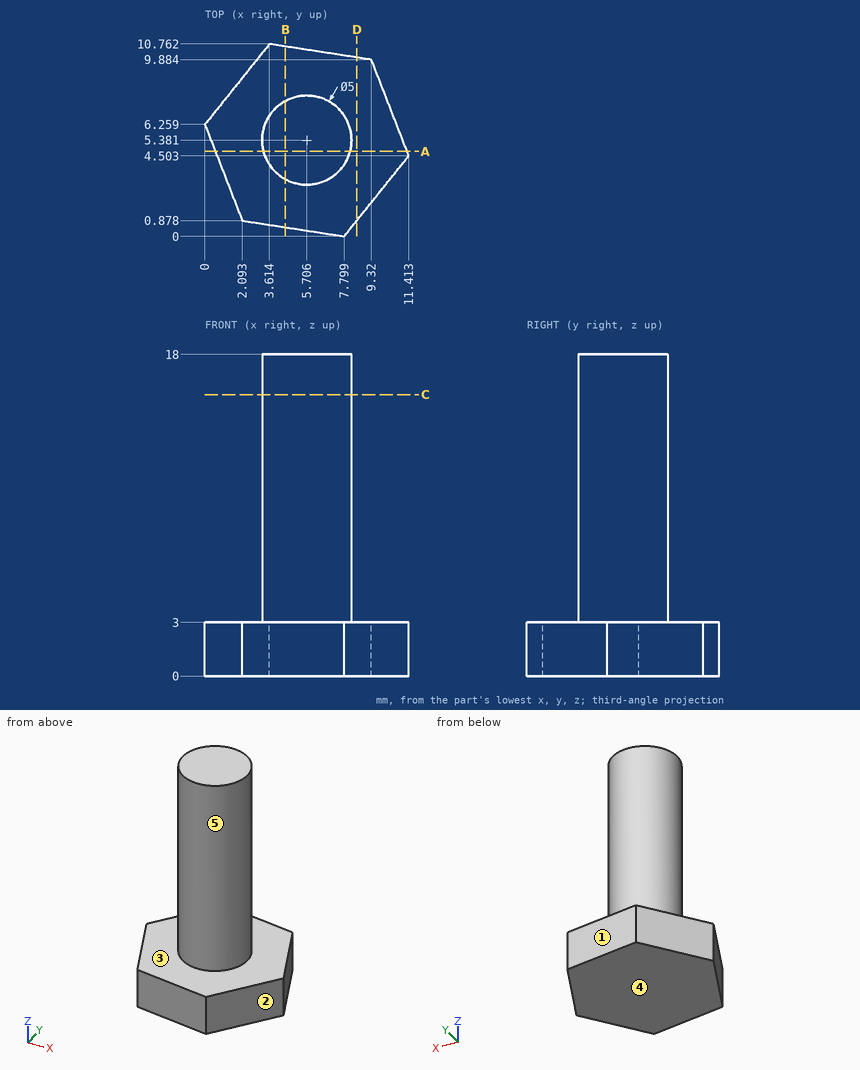
Input: dimensioned drawing with shaded views. Units: mm. Origin: part minimum x, y, z. A direction names the side the tool comes from. Round coordinates to 2 decimals unless told otherwise and drop trailing zeros. Loops run counter-clockwise (first coordinate to the right, second up) from the corner with the lowest first, then second, coordinate; pieces in that order, holes last. Notation, with made-up numbers: M -23,42 L 30,42 A18 cw 30,72 Z; hole C 88.5,78 d2. An arc over 180 degrees is marked long. Answer in a Markdown table with one row per item. Add a question column.
1. Section B-B (x = 4.5). Output: boundary loops of the cut face in (y, z) (1 decimal).
2. Mould query, pull axis Y, two halves, no side actions, for the marked faces 1, 2 and 3. Classes: released by +Y, released by -Y, zero draft, split by the parting line, or undercut.
3. Section D-D (x = 8.5). Output: boundary loops of the cut face in (y, z).
4. Ray query, probe 1 along Z at (x, y) = (9.75, 4); probe 2 along X at (y, z) = (5.5, 7.25); probe 3 along Y at (x, z) = (3.5, 7) (1 decimal). Return the intervals inside material, ascending.
5. Contact query for flat-ended pins moving along their axis: pin 1 (2 mm diameter, centred on y = 8, z = 12, fed in from +X); pin 2 (1.5 mm diameter, centred on x = 8, y = 2, fed in from +Z); pin 3 (1 mm diameter, centred on y = 1.5, z = 3, fed in from -X); pin 4 (1.5 mm diameter, centred on x = 9, z = 8, fed in from +Y). Output: stop coordinate, or through.
6. Section C-C (z = 15.75). Output: boundary loops of the cut face in (x, y), and give its area (3 significant figures).
7. Section A-A (y = 4.75). Output: boundary loops of the cut face in (x, z) (1 decimal).
8. Set-up query: the marked faces 4 and 5. Return all of +Z, -Z, +X, -X, +Y, -Y with unobstructed straight access to the full face (end or side cutting, diameter ignored); none if empty.
Values follow:
| question | item | result |
|---|---|---|
| 1 | outline | M 0.5,0 L 10.6,0 L 10.6,3 L 7.6,3 L 7.6,18 L 3.2,18 L 3.2,3 L 0.5,3 Z |
| 2 | face 1 | released by +Y |
| 2 | face 2 | released by -Y |
| 2 | face 3 | zero draft |
| 3 | outline | M 0.87,0 L 10.01,0 L 10.01,3 L 0.87,3 Z |
| 4 | probe 1 | 0 to 3 |
| 4 | probe 2 | 3.21 to 8.2 |
| 4 | probe 3 | 4.2 to 6.6 |
| 5 | pin 1 | x = 7.61 |
| 5 | pin 2 | z = 3 |
| 5 | pin 3 | x = 1.66 |
| 5 | pin 4 | through |
| 6 | outline | C 5.71,5.38 d5 |
| 6 | area | 19.6 mm^2 |
| 7 | outline | M 0.6,0 L 11.3,0 L 11.3,3 L 8.1,3 L 8.1,18 L 3.3,18 L 3.3,3 L 0.6,3 Z |
| 8 | face 4 | -Z, +X, -X, +Y, -Y |
| 8 | face 5 | +Z |
